Read the model definition and answer for the solid it produces. Units are mm, in the model's axes. Coordinates: 2 decimals unless noted, no trailing zeros. Order: outer loops, then holes, each group sorted by start corner. A loop starts at its lowest first (then second) coordinate and runs counter-clockwise, first axis right, second up. Notation, with made-up numbers: (-23, -27) - (3, -27) arc R21 ccw to (3, -18) - close; hole circle Ø3 at (2, 59). An arc over 180 degrees is marked (long way). Answer as a JSON object with one key per item and string values. Group by question number.
from build123d import *

# Parameters (mm, degrees)
F0_R     = 3
F1_DEPTH = 18
F2_DEPTH = 14


# Not quite as in the source:
# - ends of sketch curves that miss each other by under 0.0002 mm in the source are joined


with BuildPart() as f1:
    # F0 (on Front) → F1 (new body)
    with BuildSketch(Plane.XZ):
        with BuildLine():
            Line((-42.3895305789, -243.8882939158), (-24.7354158314, -250.6203213983))
            ThreePointArc((-24.7354158314, -250.6203213983), (-15.5028330705, -249.5140993631), (-11.1723924415, -241.2853938543))
            Line((-11.1723924415, -241.2853938543), (-10.5257942379, 495.2740080398))
            Line((-10.5257942379, 495.2740080398), (-87.9671722006, 524.8046568947))
            Line((-87.9671722006, 524.8046568947), (-48.8132548023, -235.0591811233))
            ThreePointArc((-48.8132548023, -235.0591811233), (-46.9127527413, -240.4278329279), (-42.3895305789, -243.8882939158))
        make_face()
        with Locations((-27.881012126, -192.8539189117)):
            Circle(F0_R, mode=Mode.SUBTRACT)
        with Locations((-30.5399937075, -49.059701124)):
            Circle(F0_R, mode=Mode.SUBTRACT)
        with Locations((-35.8245981399, 119.2769033151)):
            Circle(F0_R, mode=Mode.SUBTRACT)
        with Locations((-37.6148353963, 326.2889456799)):
            Circle(F0_R, mode=Mode.SUBTRACT)
        with BuildLine():
            ThreePointArc((-35.8713849562, 463.9863896495), (-35.6237850386, 458.3139596858), (-41.2978981422, 458.1085140717))
            Line((-41.2978981422, 458.1085140717), (-47.5773687005, 457.9045057833))
            ThreePointArc((-47.5773687005, 457.9045057833), (-53.2508540354, 457.7393262229), (-53.3777836629, 463.4137960782))
            Line((-53.3777836629, 463.4137960782), (-54.3935717097, 487.9983330149))
            ThreePointArc((-54.3935717097, 487.9983330149), (-54.636241933, 493.6693642066), (-48.9636796908, 493.8731318846))
            Line((-48.9636796908, 493.8731318846), (-42.2828997396, 494.0973559272))
            ThreePointArc((-42.2828997396, 494.0973559272), (-36.6071005964, 494.2603360531), (-36.4869165759, 488.5834695431))
            Line((-36.4869165759, 488.5834695431), (-35.8713849562, 463.9863896495))
        make_face(mode=Mode.SUBTRACT)
        with Locations((-43.7681841537, 431.407725542)):
            Circle(F0_R, mode=Mode.SUBTRACT)
        with Locations((-23.2091454593, 473.1308742023)):
            Circle(F0_R, mode=Mode.SUBTRACT)
        with Locations((-43.7681841537, 431.407725542)):
            Circle(F0_R)
        with Locations((-23.2091454593, 473.1308742023)):
            Circle(F0_R)
        with Locations((-37.6148353963, 326.2889456799)):
            Circle(F0_R)
        with Locations((-35.8245981399, 119.2769033151)):
            Circle(F0_R)
        with Locations((-27.881012126, -192.8539189117)):
            Circle(F0_R)
        with Locations((-30.5399937075, -49.059701124)):
            Circle(F0_R)
    extrude(amount=F1_DEPTH)

    # F0 (on Front) → F2 (cut)
    with BuildSketch(Plane.XZ):
        with Locations((-43.7681841537, 431.407725542)):
            Circle(F0_R)
        with Locations((-23.2091454593, 473.1308742023)):
            Circle(F0_R)
        with Locations((-37.6148353963, 326.2889456799)):
            Circle(F0_R)
        with Locations((-35.8245981399, 119.2769033151)):
            Circle(F0_R)
        with Locations((-27.881012126, -192.8539189117)):
            Circle(F0_R)
        with Locations((-30.5399937075, -49.059701124)):
            Circle(F0_R)
    extrude(amount=F2_DEPTH, mode=Mode.SUBTRACT)


solid = f1.part
1. A cutting plane is placed at A-A on y = -7.5. Write down the section's boundary in (x, z), and give its area (3 significant figures).
2. Straight lines are drawn through the part: L1, parallel to Z at x = -35, y = -12.25; L2, parallel to Z at x = -44, y = -6.25; L3, parallel to X at y = -13, z = 488. For each, find the intervals that lie inside material, in ascending order.
3. A cutting plane is placed at C-C on z = 108.5. Write down the section's boundary in (x, y), and give its area (3 significant figures).
4. A cutting plane is placed at B-B on x = -72. Write down the section's boundary in (y, z).
5. For a pull along Z with two mould halves and no side action, classify faces 1 (the flat face through (-68.664, -8.874, 150.192)), 2 (the flat face through (-53.88, -8.87, 475.53)), 3 (the flat face through (-41, -18, 142)) as pulls with the +Z half, pulls with the -Z half, needs draft (parallel to the pull), parting line crosses it, or undercut.
6. Given pin 1 (7 mm diameter, centred on x = -43.77, z = 431.41, fed in from +Y); pin 2 (3 mm diameter, centred on x = -31.5, z = -48.5, fed in from +Y); pin 3 (2 mm diameter, centred on y = -14.5, z = 267, fed in from -X); pin 4 (6 mm diameter, centred on y = -2, z = -110, fed in from +X), each flat-ended and moving along its own axis, determine where each tip first touches the part or whether it passes through.
Derived:
{
 "1": {"outline": "(-87.97, 524.8) - (-48.81, -235.06) arc R10 ccw to (-42.39, -243.89) - (-24.74, -250.62) arc R10 ccw to (-11.17, -241.29) - (-10.53, 495.27) - close; hole (-54.39, 488) - (-53.38, 463.41) arc R4 ccw (long way) to (-47.58, 457.9) - (-41.3, 458.11) arc R4 ccw (long way) to (-35.87, 463.99) - (-36.49, 488.58) arc R4 ccw (long way) to (-42.28, 494.1) - (-48.96, 493.87) arc R4 ccw (long way) to start; hole circle Ø6 at (-43.77, 431.41); hole circle Ø6 at (-37.61, 326.29); hole circle Ø6 at (-35.82, 119.28); hole circle Ø6 at (-30.54, -49.06); hole circle Ø6 at (-27.88, -192.85); hole circle Ø6 at (-23.21, 473.13)", "area": "42,200 mm2"},
 "2": {"L1": "z = -246.71 to 116.39, 122.16 to 324.82, 327.76 to 459.21, 462.85 to 504.61", "L2": "z = -243.1 to 428.42, 434.4 to 458.02, 494.04 to 508.04", "L3": "x = -86.07 to -54.4, -36.47 to -10.53"},
 "3": {"outline": "(-66.52, -18) - (-10.87, -18) - (-10.87, 0) - (-66.52, 0) - close", "area": "1,000 mm2"},
 "4": {"outline": "(-18, 214.93) - (0, 214.93) - (0, 518.72) - (-18, 518.72) - close"},
 "5": {"face 1": "pulls with the -Z half", "face 2": "undercut", "face 3": "needs draft"},
 "6": {"pin 1": "stops at y = 0", "pin 2": "stops at y = -14", "pin 3": "stops at x = -74.73", "pin 4": "stops at x = -11.05"}
}
